Part model, mm, in its own coordinate system. A direction names the side the tool comes from. Round coordinates to 2 decimals unless told otherwise and drop trailing zeros. Write each loop counter-clockwise with the first axis right and the second up, starting at its lowest first coordinate (ties: lowest second). Pieces come first, ordered by that corner, then holes. Notation, with made-up numbers: (45.5, 53.5) -> (95.5, 53.5) arc R12 cw to (95.5, 73.5) -> close; hole circle Ø10 at (33, 52). An arc over 180 degrees is marked (long way). Return JSON: item names as keys, results as strings. Group by question number.
(1) Drill centre lines: L1, parallel to Y at x = -2.25, z = 0; L2, parallel to Y at x = 6, z = 0.75; L3, parallel to Z at x = 0.75, y = 9. Where is each one in solid material? Low to high. Write a range as from..to.
(2) Saw through at C-C (y = 31). List the corners of the cut face in (x, z), plus the area to 3 significant figures.
(3) Tool access for faces 1 (the cylindrical face through (-2.95, 46.9, -12.4)), 2 (the flat face through (12.865, 21, 0)): list every direction of +Z, -Z, +X, -X, +Y, -Y with a clear straight run to the whole face (end or side of a thin tool).
(4) Drop flat-ended pins along their axis: pin 1 Ø5 at (y, z) = (15, 0) entering from +X; pin 2 Ø0.6 at (x, z) = (-11, -1.5) entering from -Y; pin 3 Ø11.5 at (y, z) = (22.5, -2) entering from +X; pin 4 Ø1 at (x, y) = (5.5, 72) entering from +Z. Give the stop position or say it passes through.
(5) Saw through at B-B (y = 15). List the corners of the cut face in (x, z).
(6) Saw through at A-A (z = 0). List the corners of the cut face in (x, y), plus the area to 3 significant figures.
(7) Mould opens along Y. For faces 3 (the flat face through (-10.757, 21, 0)), 4 (the flat face through (1, 0, 0)), 5 (the cylindrical face through (1.14, 76.12, 0.54)) say: +Y half, -Y half, draft (parallel to the pull), parting line (faces both ways), or undercut.
(8) Saw through at D-D (x = 10.25). State how many separate pieces and enclosed holes the cut face has, plus the area to 3 significant figures.
from build123d import *

# Parameters (mm, degrees)
SKETCH_1_R          = 13
EXTRUDE_1_DEPTH     = 90
FILLET_1_R          = 5
SKETCH_3_R          = 4
CUT_EXTRUDE_2_DEPTH = 20
SKETCH_4_W          = 5.638292822
SKETCH_4_H          = 34.801876381
CUT_EXTRUDE_3_DEPTH = 22.5
SKETCH_5_R          = 2.5
CUT_EXTRUDE_1_DEPTH = 55


with BuildPart() as part:
    # Эскиз1 → Вытянуть1 (new body)
    with BuildSketch(Plane(origin=(0, 0, 0), x_dir=(1, 0, 0), z_dir=(0, 1, 0))):
        with Locations(Location((0.959256222, 0, 0), (0, 0, 90))):
            Circle(SKETCH_1_R)
    extrude(amount=EXTRUDE_1_DEPTH)

    # Скругление1
    fillet_1_edges = [part.edges().sort_by_distance(p)[0] for p in [
        (0.959256222, 0, 13),
    ]]
    fillet(fillet_1_edges, radius=FILLET_1_R)

    # Эскиз3 → Вытянуть2 (cut, symmetric)
    with BuildSketch(Plane(origin=(0, 0, 0), x_dir=(0, 0, -1), z_dir=(1, 0, 0))):
        with Locations((0, 15)):
            Circle(SKETCH_3_R)
    extrude(amount=CUT_EXTRUDE_2_DEPTH, both=True, mode=Mode.SUBTRACT)

    # Эскиз4 → Вытянуть3 (cut, symmetric)
    with BuildSketch(Plane.XY):
        with Locations((-13.576502311, 16.48112444)):
            Rectangle(SKETCH_4_W, SKETCH_4_H)
        with Locations((15.684293194, 16.48112444)):
            Rectangle(SKETCH_4_W, SKETCH_4_H)
    extrude(amount=CUT_EXTRUDE_3_DEPTH, both=True, mode=Mode.SUBTRACT)

    # Эскиз5 → Вырез-Вытянуть1 (cut, symmetric)
    with BuildSketch(Plane(origin=(0, 0, 0), x_dir=(0, 0, -1), z_dir=(1, 0, 0))):
        with Locations((9.34e-07, 78.55964506)):
            Circle(SKETCH_5_R)
    extrude(amount=CUT_EXTRUDE_1_DEPTH, both=True, mode=Mode.SUBTRACT)


solid = part.part
Computed values:
{
 "1": {"L1": "0..11, 19..76.06, 81.06..90", "L2": "0..11.07, 18.93..76.17, 80.94..90", "L3": "-13..13"},
 "2": {"outline": "(-10.76, -5.63) arc R13 ccw to (12.87, -5.22) -> (12.87, 5.22) arc R13 ccw to (-10.76, 5.63) -> close", "area": "514 mm2"},
 "3": {"face 1": "+Y, -Y", "face 2": "+Z, -Z, +X, -Y"},
 "4": {"pin 1": "through", "pin 2": "y = 1.7", "pin 3": "x = 12.87", "pin 4": "z = 12.36"},
 "5": {"outline": "(-10.76, -5.63) arc R13 ccw to (12.87, -5.22) -> (12.87, -4) -> (-10.76, -4) -> close; (-10.76, 4) -> (12.87, 4) -> (12.87, 5.22) arc R13 ccw to (-10.76, 5.63) -> close"},
 "6": {"outline": "(-12.04, 33.88) -> (-10.76, 33.88) -> (-10.76, 19) -> (12.87, 19) -> (12.87, 33.88) -> (13.96, 33.88) -> (13.96, 76.06) -> (-12.04, 76.06) -> close; (-12.04, 81.06) -> (13.96, 81.06) -> (13.96, 90) -> (-12.04, 90) -> close; (-10.76, 1.66) arc R5 ccw to (-7.04, 0) -> (8.96, 0) arc R5 ccw to (12.87, 1.88) -> (12.87, 11) -> (-10.76, 11) -> close", "area": "1,940 mm2"},
 "7": {"face 3": "draft", "face 4": "-Y half", "face 5": "undercut"},
 "8": {"separate pieces": "1", "enclosed holes": "2", "area": "1,550 mm2"}
}
